from build123d import *

# Parameters (mm, degrees)
SKETCH1_W           = 245
SKETCH1_H           = 70
BOSS_EXTRUDE1_DEPTH = 3
SKETCH2_R           = 10
CUT_EXTRUDE1_DEPTH  = 3


with BuildPart() as part:
    # Sketch1 → Boss-Extrude1 (new body)
    with BuildSketch(Plane.XY):
        Rectangle(SKETCH1_W, SKETCH1_H)
    extrude(amount=BOSS_EXTRUDE1_DEPTH)

    # Sketch2 → Cut-Extrude1 (cut)
    with BuildSketch(Plane.XY.offset(3)):
        with Locations((-80, 0)):
            Circle(SKETCH2_R)
        Circle(SKETCH2_R)
        with Locations((80, 0)):
            Circle(SKETCH2_R)
    extrude(amount=-CUT_EXTRUDE1_DEPTH, mode=Mode.SUBTRACT)


solid = part.part
The listing builds one solid part. Answer for the finished solid, in the listing's coordinates (mm). Give positions to 0.01 mm unless a question says otherwise; leave off trailing zeros. Write each loop counter-clockwise with the first axis right and the second up, starting at its lowest first coordinate (ties: lowest second). Pieces come first, ordered by that corner, then holes.
Item 1: Section A-A, the plane y = 0 is taken. Write down the section's boundary in (x, z), plus the area to 3 significant figures.
Item 2: Section C-C, the plane x = -80 is taken. Write down the section's boundary in (y, z).
Item 3: Determine the mould class of faces 1 (the cylindrical face through (-2.17, -9.76, 1.52)), 2 (the flat face through (-2, 16, 0)) for opening direction Y: released by +Y, released by -Y, zero draft, split by the parting line, or undercut.
Item 4: Find the intervals of material crossed by line 1 along Y through (x, z) = (80, 2.15); line 2 along X through (y, z) = (-2, 0.65); line 3 along Y through (x, z) = (-85.5, 2.7), in increasing order.
Item 5: Section D-D, the plane x = 75.5 is taken. Write down the section's boundary in (y, z), plus the area to 3 significant figures.
Item 6: Section B-B, the plane z = 2.1 is taken. Write down the section's boundary in (x, y), plus the area to 3 significant figures.
Completed:
1. outline: (-122.5, 0) - (-90, 0) - (-90, 3) - (-122.5, 3) - close; (-70, 0) - (-10, 0) - (-10, 3) - (-70, 3) - close; (10, 0) - (70, 0) - (70, 3) - (10, 3) - close; (90, 0) - (122.5, 0) - (122.5, 3) - (90, 3) - close
1. area: 555 mm2
2. outline: (-35, 0) - (-10, 0) - (-10, 3) - (-35, 3) - close; (10, 0) - (35, 0) - (35, 3) - (10, 3) - close
3. face 1: undercut
3. face 2: zero draft
4. line 1: y = -35 to -10, 10 to 35
4. line 2: x = -122.5 to -89.8, -70.2 to -9.8, 9.8 to 70.2, 89.8 to 122.5
4. line 3: y = -35 to -8.35, 8.35 to 35
5. outline: (-35, 0) - (-8.93, 0) - (-8.93, 3) - (-35, 3) - close; (8.93, 0) - (35, 0) - (35, 3) - (8.93, 3) - close
5. area: 156 mm2
6. outline: (-122.5, -35) - (122.5, -35) - (122.5, 35) - (-122.5, 35) - close; hole circle Ø20 at (-80, 0); hole circle Ø20 at (0, 0); hole circle Ø20 at (80, 0)
6. area: 16,200 mm2
